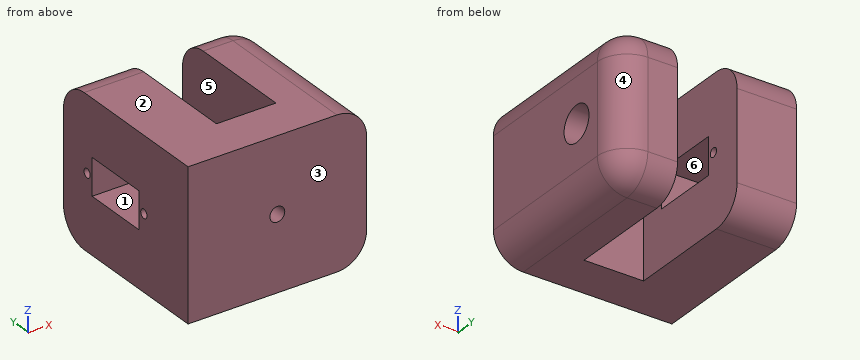
```python
from build123d import *

# Parameters (mm, degrees)
SKETCH1_W           = 60
SKETCH1_H           = 50
BOSS_EXTRUDE1_DEPTH = 15
SKETCH5_W           = 20
SKETCH5_H           = 50
BOSS_EXTRUDE5_DEPTH = 45
SKETCH6_R           = 6
CUT_EXTRUDE1_DEPTH  = 84
SKETCH7_R           = 2.5
CUT_EXTRUDE2_DEPTH  = 19
FILLET1_R           = 10
FILLET3_R           = 10
SKETCH8_R           = 6
SKETCH8_R_2         = 1.5
CUT_EXTRUDE3_DEPTH  = 30


with BuildPart() as part:
    # Sketch1 → Boss-Extrude1 (new body)
    with BuildSketch(Plane(origin=(0, 0, 0), x_dir=(1, 0, 0), z_dir=(0, 1, 0))):
        with Locations((30, -25)):
            Rectangle(SKETCH1_W, SKETCH1_H)
    extrude(amount=BOSS_EXTRUDE1_DEPTH)

    # Sketch5 → Boss-Extrude5 (add)
    with BuildSketch(Plane(origin=(0, 15, 0), x_dir=(1, 0, 0), z_dir=(0, 1, 0))):
        with Locations((10, -25)):
            Rectangle(SKETCH5_W, SKETCH5_H)
        with Locations((50, -25)):
            Rectangle(SKETCH5_W, SKETCH5_H)
    extrude(amount=BOSS_EXTRUDE5_DEPTH)

    # Sketch6 → Cut-Extrude1 (cut)
    with BuildSketch(Plane.ZY):
        with Locations((25, 40)):
            Circle(SKETCH6_R)
    extrude(amount=-CUT_EXTRUDE1_DEPTH, mode=Mode.SUBTRACT)

    # Sketch7 → Cut-Extrude2 (cut)
    with BuildSketch(Plane.XZ):
        with Locations((30, 25)):
            Circle(SKETCH7_R)
    extrude(amount=-CUT_EXTRUDE2_DEPTH, mode=Mode.SUBTRACT)

    # Fillet1
    fillet1_edges = [part.edges().sort_by_distance(p)[0] for p in [
        (10, 60, 50),
        (10, 60, 0),
        (50, 60, 0),
        (50, 60, 50),
    ]]
    fillet(fillet1_edges, radius=FILLET1_R)

    # Fillet3
    fillet3_edges = [part.edges().sort_by_distance(p)[0] for p in [
        (60, 25, 50),
        (60, 60, 25),
        (60, 25, 0),
        (60, 57.071067812, 2.928932188),
        (60, 57.071067812, 47.071067812),
    ]]
    fillet(fillet3_edges, radius=FILLET3_R)

    # Sketch8 → Cut-Extrude3 (cut)
    with BuildSketch(Plane.ZY):
        Polygon((31.2, 46.2), (25, 46.2), (18.8, 46.2), (18.8, 23.7), (25, 23.7), (31.2, 23.7), align=None)
        with Locations((25, 40)):
            Circle(SKETCH8_R, mode=Mode.SUBTRACT)
        with Locations((25, 48.6)):
            Circle(SKETCH8_R_2)
        with Locations((25, 21.3)):
            Circle(SKETCH8_R_2)
    extrude(amount=-CUT_EXTRUDE3_DEPTH, mode=Mode.SUBTRACT)


solid = part.part
```
Here's how the part is built. I have some questions about the finished solid (model axes, mm). Face numbers are marked on the shaded views. A direction names the side the tool comes from. Give positions to 0.01 mm unless a question says otherwise; leave off trailing zeros. Write each loop counter-clockwise with the first axis right and the second up, starting at its lowest first coordinate (ties: lowest second). Pieces come first, ordered by that corner, then holes. Notation, with made-up numbers: (-18, -29.75) -> (30, -29.75) arc R32 cw to (30, 7.25) -> close; hole circle Ø10 at (43, 19). An arc over 180 degrees is marked (long way). Write each question's results on one line, items separated by ' | '.
Item 1: On a 3-axis mill with a long thin cutter (end or side, diameter ignored), from which of +Z, -Z, +X, -X, +Y, -Y can I reach the whole of each face in a straight line? I mean the marked faces 4, 5 and 6. Say none if no direction works.
Output:
face 4: +Z, -Z, +X, +Y | face 5: +Z, -Z, +Y | face 6: -X
Item 2: Suppose I cut it at D-D on y = 40. Write out the boundary of the cut face in (x, z), plus the area to 3 significant figures.
Output:
outline: (0, 0) -> (20, 0) -> (20, 18.8) -> (0, 18.8) -> close; (0, 31.2) -> (20, 31.2) -> (20, 50) -> (0, 50) -> close; (40, 0) -> (50, 0) arc R10 ccw to (60, 10) -> (60, 19) -> (40, 19) -> close; (40, 31) -> (60, 31) -> (60, 40) arc R10 ccw to (50, 50) -> (40, 50) -> close | area: 1,470 mm^2
Item 3: For pin 1 Ø8 at (x, z) = (30, 25) entering from +Y; pin 2 Ø7 at (y, z) = (40, 25) entering from +X; pin 3 Ø2.5 at (y, z) = (21.3, 25) entering from -X, each with a flat end and sliding along its axis, tell me the tip position at first contact or that it passes through.
Output:
pin 1: stops at y = 15 | pin 2: passes through | pin 3: stops at x = 40
Item 4: Suppose I cut it at C-C on z = 25. Give the number of separate pieces and of enclosed holes in the cut face, plus the area to 3 significant figures.
Output:
separate pieces: 6 | enclosed holes: 0 | area: 1,790 mm^2
Item 5: If I drill on L1, parallel to Y at x = 10, z = 25; L2, parallel to X at y = 41, z = 40.5; L3, parallel to Z at x = 15.5, y = 29, over which ranges is the centre line in solid material (lowest first)?
Output:
L1: y = 0 to 19.8, 22.8 to 23.7, 46.2 to 47.1, 50.1 to 60 | L2: x = 0 to 20, 40 to 59.99 | L3: z = 0 to 18.8, 31.2 to 50
Item 6: We'd pull the mould along Z, two halves only. Please class the marked faces 1, 2 and 3: pulls with the +Z half, pulls with the -Z half, needs draft (parallel to the pull), parting line crosses it, or undercut.
Output:
face 1: undercut | face 2: pulls with the +Z half | face 3: needs draft
Item 7: Suppose I cut it at A-A on x = 30. Write out the boundary of the cut face in (y, z).
Output:
outline: (0, 0) -> (15, 0) -> (15, 22.5) -> (0, 22.5) -> close; (0, 27.5) -> (15, 27.5) -> (15, 50) -> (0, 50) -> close
Item 8: Suppose I cut it at B-B on y = 48.6. Write out the boundary of the cut face in (x, z), plus the area to 3 significant figures.
Output:
outline: (0, 0) -> (20, 0) -> (20, 23.5) -> (0, 23.5) -> close; (0, 26.5) -> (20, 26.5) -> (20, 50) -> (0, 50) -> close; (40, 0) -> (50, 0) arc R10 ccw to (60, 10) -> (60, 40) arc R10 ccw to (50, 50) -> (40, 50) -> close | area: 1,900 mm^2
